```python
from build123d import *

# Parameters (mm, degrees)
F0_W        = 182.7820166945
F0_H        = 5.2849859931
F1_DEPTH    = 20
F2_T1_DEPTH = 45
F3_D        = 2
F4_T1_DEPTH = 45
F5_D        = 2
F6_W        = 10.6622725725
F6_H        = 5.6903085506
F9_DEPTH    = 18
F6_W_2      = 10.1688206196
F6_H_2      = 8.087759139
F10_DEPTH   = 18


# Not quite as in the source:
# - a fillet or chamfer that OpenCascade refuses, or shapes differently, is made with other operations: its cross-section is extruded or revolved along the edge and cut away or added


with BuildPart() as f1:
    # F0 (on Front) → F1 (new body)
    with BuildSketch(Plane.XZ):
        with Locations((16.4561159909, 2.6424929965)):
            Rectangle(F0_W, F0_H)
    extrude(amount=-F1_DEPTH)

    # F2: fillet of radius 5 on 2 edges, made by hand

    # F2_s2 → F2_t1 (cut)
    with BuildSketch(Plane.XZ.offset(-32.5)):
        with BuildLine():
            ThreePointArc((-74.9348923564, 0.2849859931), (-73.4704262623, 3.820519899), (-69.9348923564, 5.2849859931))
            Line((-69.9348923564, 5.2849859931), (-74.9348923564, 5.2849859931))
            Line((-74.9348923564, 5.2849859931), (-74.9348923564, 0.2849859931))
        make_face()
        with BuildLine():
            ThreePointArc((-74.9348923564, 5), (-73.4704262623, 1.4644660941), (-69.9348923564, 0))
            Line((-69.9348923564, 0), (-74.9348923564, 0))
            Line((-74.9348923564, 0), (-74.9348923564, 5))
        make_face()
    extrude(amount=F2_T1_DEPTH, mode=Mode.SUBTRACT)

    # F3 (through all)
    with Locations(Plane.XZ):
        with Locations((-69.9340328574, 2.630488947)):
            Hole(F3_D / 2)

    # F4: fillet of radius 5 on 2 edges, made by hand

    # F4_s2 → F4_t1 (cut)
    with BuildSketch(Plane.XZ.offset(-32.5)):
        with BuildLine():
            ThreePointArc((102.8471243382, 5.2849859931), (106.3826582441, 3.820519899), (107.8471243382, 0.2849859931))
            Line((107.8471243382, 0.2849859931), (107.8471243382, 5.2849859931))
            Line((107.8471243382, 5.2849859931), (102.8471243382, 5.2849859931))
        make_face()
        with BuildLine():
            ThreePointArc((107.8471243382, 5), (106.3826582441, 1.4644660941), (102.8471243382, 0))
            Line((102.8471243382, 0), (107.8471243382, 0))
            Line((107.8471243382, 0), (107.8471243382, 5))
        make_face()
    extrude(amount=F4_T1_DEPTH, mode=Mode.SUBTRACT)

    # F5 (through all)
    with Locations(Plane.XZ):
        with Locations((102.8473824263, 2.641917672)):
            Hole(F5_D / 2)


with BuildPart() as f1_1:
    # F7: moved
    add(f1.part.moved(Location((-1, 1, 0))))


with BuildPart() as f1_2:
    # F8: moved
    add(f1_1.part.moved(Location((0, -2, 0))))

    # F6 (on Front) → F9 (cut)
    with BuildSketch(Plane.XZ):
        with Locations((-71.0640922189, 2.8451542753)):
            Rectangle(F6_W, F6_H)
    extrude(amount=-F9_DEPTH, mode=Mode.SUBTRACT)

    # F6 (on Front) → F10 (cut)
    with BuildSketch(Plane.XZ):
        with Locations((102.1384820342, 2.511022496)):
            Rectangle(F6_W_2, F6_H_2)
    extrude(amount=-F10_DEPTH, mode=Mode.SUBTRACT)


solid = f1_2.part
```
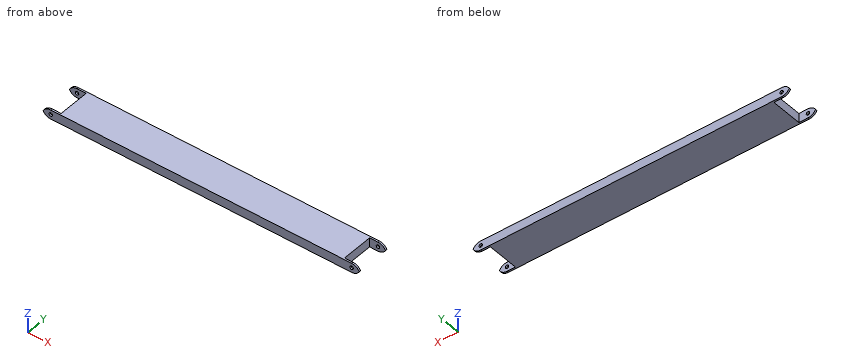
Design review of the part built by this model. Coordinates are the model's own, in mm. Coordinates: 2 decimals unless noted, no trailing zeros. Order: outer loops, then holes, each group sorted by start corner. A loop starts at its lowest first (then second) coordinate and runs counter-clockwise, first axis right, second up. Notation, with made-up numbers: (25.5, 56) - (47.5, 56) arc R21 cw to (47.5, 78) - close; hole circle Ø11 at (-18, -7). An arc over 180 degrees is marked (long way). Answer in a Markdown table with one row per item.
(1) Wall thickness on line 1 along X through (y, z) = (2.5, 4.75); line 2 along Y through (x, z) = (-66.5, 3.8): over which ranges is each line inside the solid? List them lowest first. Write a range as from..to.
Checked values:
| item | result |
|---|---|
| line 1 | -65.73..97.05 |
| line 2 | -1..0, 18..19 |
(2) Clearance check with flat-ended pins moving along their axes: pin 1 (2.5 mm diameter, centred on y = 10, z = 3.5, fed in from -X); pin 2 (1.6 mm diameter, centred on x = -71, z = 2.5, fed in from -Y); pin 3 (1 mm diameter, centred on y = 2, z = 2, fed in from +X). State where each tip first meets the part, or that it passes through.
Checked values:
| item | result |
|---|---|
| pin 1 | x = -65.73 |
| pin 2 | through |
| pin 3 | x = 97.05 |
(3) Consider section A-A on y = 14.25. State the section outline as (x, z) points, plus the area to 3 significant figures.
Checked values:
| item | result |
|---|---|
| outline | (-65.73, 0) - (97.05, 0) - (97.05, 5.28) - (-65.73, 5.28) - close |
| area | 860 mm^2 |
